```python
from build123d import *

# Parameters (mm, degrees)
F0_R     = 20
F1_DEPTH = 12.5
F2_R     = 2.5
F3_R     = 2.5
F4_R     = 15
F5_DEPTH = 2.5


with BuildPart() as f1:
    # F0 (on Top) → F1 (new body)
    with BuildSketch(Plane.XY):
        Circle(F0_R)
    extrude(amount=F1_DEPTH)

    # F2
    f2_edges = [f1.edges().sort_by_distance(p)[0] for p in [
        (-20, 0, 12.5),
    ]]
    fillet(f2_edges, radius=F2_R)

    # F3
    f3_edges = [f1.edges().sort_by_distance(p)[0] for p in [
        (-20, 0, 0),
    ]]
    fillet(f3_edges, radius=F3_R)

    # F4 (on face) → F5 (cut)
    with BuildSketch(Plane.XY.offset(12.5)):
        Circle(F4_R)
        with BuildLine():
            Line((-3.75, 3.75), (-3.75, 11.92424))
            ThreePointArc((-3.75, 11.92424), (0, 12.5), (3.75, 11.92424))
            Line((3.75, 11.92424), (3.75, 3.75))
            Line((3.75, 3.75), (11.92424, 3.75))
            ThreePointArc((11.92424, 3.75), (12.5, 0), (11.92424, -3.75))
            Line((11.92424, -3.75), (3.75, -3.75))
            Line((3.75, -3.75), (3.75, -11.92424))
            ThreePointArc((3.75, -11.92424), (0, -12.5), (-3.75, -11.92424))
            Line((-3.75, -11.92424), (-3.75, -3.75))
            Line((-3.75, -3.75), (-11.92424, -3.75))
            ThreePointArc((-11.92424, -3.75), (-12.5, 0), (-11.92424, 3.75))
            Line((-11.92424, 3.75), (-3.75, 3.75))
        make_face(mode=Mode.SUBTRACT)
    extrude(amount=-F5_DEPTH, mode=Mode.SUBTRACT)


solid = f1.part
```
Design review of the part built by this model. Coordinates are the model's own, in mm. A direction names the side the tool comes from. Give positions to 0.01 mm unless a question says otherwise; leave off trailing zeros. Order: outer loops, then holes, each group sorted by start corner. A loop starts at its lowest first (then second) coordinate and runs counter-clockwise, first axis right, second up. Notation, with made-up numbers: (14.5, 0) -> (57.5, 0) arc R38 ccw to (57.5, 39) -> close; hole circle Ø3 at (70.25, -24). An arc over 180 degrees is marked (long way). Write each question's results on one line, items separated by ' | '. Start each with the question number.
Q1. Add section B-B on y = 0. Give the boundary of the cut face in (x, z).
Q2. Add section A-A on z = 11. Give the boundary of the cut face in (x, y).
Q3. Machinability: for faces 1 (the flat face through (0, 0, 12.5)), 2 (the flat face through (3.75, 8, 11)), which of the approach directions +Z, -Z, +X, -X, +Y, -Y give a long, thin tool a straight path to every point of the face, cutting with its end or side? Answer none if there is none.
Q4. Mouldability with a two-part tool opening along X and no side actions: class faces 3 (the cylindrical face through (-4.336, -19.524, 6.198)), 4 (the flat face through (0, 0, 0)), 5 (the flat face through (8, 3.75, 11)) as +X half, -X half, draft (parallel to the pull), parting line (faces both ways), or undercut.
Q5. Wall thickness on L1, parallel to Y at x = 0, z = 11.8; L2, parallel to Y at x = 0, z = 10.7; L3, parallel to X at y = 9, z = 11.75: over which ranges is each line inside the solid? List them lowest first. Write a range as from..to.
Q6. Add section D-D on z = 3. Give the boundary of the cut face in (x, y).
Q7. For pin 1 (3 mm diameter, centred on x = 1.5, z = 2, fed in from +Y); pin 2 (1.2 mm diameter, centred on y = -6.5, z = 11, fed in from -X); pin 3 (3 mm diameter, centred on x = -7.5, z = 11, fed in from -Y), all flat-tipped, find the tip position at first contact; note any pin that passes through.
Found:
1) outline: (-20, 2.5) arc R2.5 ccw to (-17.5, 0) -> (17.5, 0) arc R2.5 ccw to (20, 2.5) -> (20, 10) arc R2.5 ccw to (17.5, 12.5) -> (15, 12.5) -> (15, 10) -> (12.5, 10) -> (12.5, 12.5) -> (-12.5, 12.5) -> (-12.5, 10) -> (-15, 10) -> (-15, 12.5) -> (-17.5, 12.5) arc R2.5 ccw to (-20, 10) -> close
2) outline: circle Ø39.58 at (0, 0); (-11.92, -3.75) -> (-3.75, -3.75) -> (-3.75, -11.92) arc R12.5 ccw to (3.75, -11.92) -> (3.75, -3.75) -> (11.92, -3.75) arc R12.5 ccw to (11.92, 3.75) -> (3.75, 3.75) -> (3.75, 11.92) arc R12.5 ccw to (-3.75, 11.92) -> (-3.75, 3.75) -> (-11.92, 3.75) arc R12.5 ccw to start; hole circle Ø30 at (0, 0)
3) face 1: +Z, +X, -X, +Y, -Y | face 2: +Z
4) face 3: parting line | face 4: draft | face 5: undercut
5) L1: y = -19.23..-15, -12.5..12.5, 15..19.23 | L2: y = -19.9..-15, -12.5..12.5, 15..19.9 | L3: x = -17.06..-12, -3.75..3.75, 12..17.06
6) outline: circle Ø40 at (0, 0)
7) pin 1: stops at y = 20 | pin 2: stops at x = -18.99 | pin 3: stops at y = -19.01
